from build123d import *

# Parameters (mm, degrees)
SKETCH_1_W      = 15
SKETCH_1_H      = 32
SKETCH_1_R      = 2.5
SKETCH_1_W_2    = 10
SKETCH_1_H_2    = 15
EXTRUDE_1_DEPTH = 5
FILLET_1_R      = 3


with BuildPart() as part:
    # 草图1 → 凸台-拉伸1 (new body)
    with BuildSketch(Plane.XY):
        with Locations((0, 12.5)):
            Rectangle(SKETCH_1_W, SKETCH_1_H)
        with Locations((0, 25)):
            Circle(SKETCH_1_R, mode=Mode.SUBTRACT)
        Circle(SKETCH_1_R, mode=Mode.SUBTRACT)
        with Locations((0, 12.5)):
            Rectangle(SKETCH_1_W_2, SKETCH_1_H_2, mode=Mode.SUBTRACT)
    extrude(amount=EXTRUDE_1_DEPTH)

    # 圆角1
    fillet_1_edges = [part.edges().sort_by_distance(p)[0] for p in [
        (5, 5, 2.5),
        (5, 20, 2.5),
        (-5, 20, 2.5),
        (-5, 5, 2.5),
        (7.5, -3.5, 2.5),
        (-7.5, -3.5, 2.5),
        (-7.5, 28.5, 2.5),
        (7.5, 28.5, 2.5),
    ]]
    fillet(fillet_1_edges, radius=FILLET_1_R)


solid = part.part
Work out the finished part from the listing and answer in its coordinate system (mm). A direction names the side the tool comes from. Give positions to 0.01 mm unless a question says otherwise; leave off trailing zeros. Write each loop counter-clockwise with the first axis right and the second up, starting at its lowest first coordinate (ties: lowest second). Pieces come first, ordered by that corner, then holes. Notation, with made-up numbers: (32, -6.5) - (86, -6.5) arc R30 ccw to (86, 31.5) - close; hole circle Ø8 at (75.5, 5). An arc over 180 degrees is marked (long way). One line per item, written item: value. Start each with the question number.
1. Consider probe 1 along Y at (x, z) = (0, 1.15); probe 2 along Y at (x, z) = (-1.25, 0.8); probe 3 along X at (y, z) = (11, 2). Determine where each line is inside the solid, lowest interval first.
2. Find section A-A (x = 1.5). Write down the section's boundary in (y, z).
3. For a pull along X with two mould halves and no side action, classify faces 1 (the flat face through (-7.5, 12, 2)), 2 (the cylindrical face through (-4.1, 19.14, 2.54)), 3 (the flat face through (0, -3.5, 2)) as +X half, -X half, draft (parallel to the pull), parting line (faces both ways), or undercut.
4. Find section B-B (y = 25). Write down the section's boundary in (x, z), then the cut area to 3 significant figures.
5. Find section D-D (x = 0). Write down the section's boundary in (y, z), then the cut area to 3 significant figures.
6. Given pin 1 (6.5 mm diameter, centred on x = 0, y = 0, fed in from -Z), flat-ended and moving along its own axis, determine where the tip first touches the part or whether it passes through.
7. For faces 4 (the flat face through (-7, 13, 0)), 5 (the cylindrical face through (4.14, 19.1, 2.54)), determine the directions among +Z, -Z, +X, -X, +Y, -Y from which every point of the face is accessible in a straight line to the end or side of a thin tool.
8. Find section C-C (z = 2). Write down the section's boundary in (x, y).
Geometry results:
1. probe 1: -3.5 to -2.5, 2.5 to 5, 20 to 22.5, 27.5 to 28.5
1. probe 2: -3.5 to -2.17, 2.17 to 5, 20 to 22.83, 27.17 to 28.5
1. probe 3: -7.5 to -5, 5 to 7.5
2. outline: (-3.5, 0) - (-2, 0) - (-2, 5) - (-3.5, 5) - close; (2, 0) - (5, 0) - (5, 5) - (2, 5) - close; (20, 0) - (23, 0) - (23, 5) - (20, 5) - close; (27, 0) - (28.5, 0) - (28.5, 5) - (27, 5) - close
3. face 1: -X half
3. face 2: undercut
3. face 3: draft
4. outline: (-7.5, 0) - (-2.5, 0) - (-2.5, 5) - (-7.5, 5) - close; (2.5, 0) - (7.5, 0) - (7.5, 5) - (2.5, 5) - close
4. area: 50.0 mm2
5. outline: (-3.5, 0) - (-2.5, 0) - (-2.5, 5) - (-3.5, 5) - close; (2.5, 0) - (5, 0) - (5, 5) - (2.5, 5) - close; (20, 0) - (22.5, 0) - (22.5, 5) - (20, 5) - close; (27.5, 0) - (28.5, 0) - (28.5, 5) - (27.5, 5) - close
5. area: 35.0 mm2
6. pin 1: z = 0
7. face 4: -Z, +X, -X, +Y, -Y
7. face 5: +Z, -Z
8. outline: (-7.5, -0.5) arc R3 ccw to (-4.5, -3.5) - (4.5, -3.5) arc R3 ccw to (7.5, -0.5) - (7.5, 25.5) arc R3 ccw to (4.5, 28.5) - (-4.5, 28.5) arc R3 ccw to (-7.5, 25.5) - close; hole (-5, 8) arc R3 ccw to (-2, 5) - (2, 5) arc R3 ccw to (5, 8) - (5, 17) arc R3 ccw to (2, 20) - (-2, 20) arc R3 ccw to (-5, 17) - close; hole circle Ø5 at (0, 0); hole circle Ø5 at (0, 25)
